Can you work these out from the model? Positions are in its coordinate system, mm. A direction names the side the tool comes from. Give positions to 0.01 mm unless a question says otherwise; leave off trailing zeros. Order: outer loops, then holes, each group sorted by start corner. A loop starts at its lowest first (then second) coordinate and runs counter-clockwise, first axis right, second up. Notation, with made-up numbers: (67.25, 33.25) - (96.25, 33.25) arc R29 ccw to (96.25, 63.25) - close; hole circle Ø8 at (61, 14.25). An arc over 180 degrees is marked (long way). Answer as a JSON object with one key per item and string values.
```python
from build123d import *

# Parameters (mm, degrees)
F0_R     = 32.6
F0_R_2   = 4.75
F1_DEPTH = 29.6
F2_R     = 2.45
F3_DEPTH = 25


with BuildPart() as f1:
    # F0 (on Front) → F1 (new body)
    with BuildSketch(Plane.XZ):
        Circle(F0_R)
        with BuildLine():
            ThreePointArc((13.747567, 17.874756), (15.860659, 16.029411), (17.728264, 13.935967))
            ThreePointArc((17.728264, 13.935967), (21.3105, 7.373268), (22.55, 0))
            ThreePointArc((22.55, 0), (22.22215, -3.831257), (21.248135, -7.55111))
            ThreePointArc((21.248135, -7.55111), (20.146089, -10.131023), (18.732227, -12.55413))
            ThreePointArc((18.732227, -12.55413), (10.343662, -20.037743), (-0.615498, -22.541598))
            ThreePointArc((-0.615498, -22.541598), (-3.409691, -22.290727), (-6.151111, -21.694846))
            ThreePointArc((-6.151111, -21.694846), (-15.860659, -16.029411), (-21.628533, -6.380364))
            ThreePointArc((-21.628533, -6.380364), (-22.253394, -3.645404), (-22.533822, -0.854022))
            ThreePointArc((-22.533822, -0.854022), (-20.146089, 10.131023), (-12.751671, 18.598317))
            ThreePointArc((-12.751671, 18.598317), (-10.343662, 20.037743), (-7.775557, 21.167031))
            ThreePointArc((-7.775557, 21.167031), (3.409691, 22.290727), (13.747567, 17.874756))
        make_face(mode=Mode.SUBTRACT)
        with BuildLine():
            ThreePointArc((-5.174181, 7.546545), (-4.197096, 8.130614), (-3.155049, 8.58884))
            Line((-3.155049, 8.58884), (-7.775557, 21.167031))
            ThreePointArc((-7.775557, 21.167031), (-10.343662, 20.037743), (-12.751671, 18.598317))
            Line((-12.751671, 18.598317), (-5.174181, 7.546545))
        make_face()
        with BuildLine():
            ThreePointArc((5.578281, 7.25295), (6.4357, 6.504173), (7.193508, 5.654727))
            Line((7.193508, 5.654727), (17.728264, 13.935967))
            ThreePointArc((17.728264, 13.935967), (15.860659, 16.029411), (13.747567, 17.874756))
            Line((13.747567, 17.874756), (5.578281, 7.25295))
        make_face()
        with BuildLine():
            Line((21.248135, -7.55111), (8.621749, -3.063976))
            ThreePointArc((8.621749, -3.063976), (8.174577, -4.110814), (7.600881, -5.094026))
            Line((7.600881, -5.094026), (18.732227, -12.55413))
            ThreePointArc((18.732227, -12.55413), (20.146089, -10.131023), (21.248135, -7.55111))
        make_face()
        with BuildLine():
            Line((-0.615498, -22.541598), (-0.249747, -9.146591))
            ThreePointArc((-0.249747, -9.146591), (-1.383533, -9.044796), (-2.495905, -8.803008))
            Line((-2.495905, -8.803008), (-6.151111, -21.694846))
            ThreePointArc((-6.151111, -21.694846), (-3.409691, -22.290727), (-0.615498, -22.541598))
        make_face()
        with BuildLine():
            ThreePointArc((-8.776101, -2.588928), (-9.029648, -1.479177), (-9.143436, -0.346532))
            Line((-9.143436, -0.346532), (-22.533822, -0.854022))
            ThreePointArc((-22.533822, -0.854022), (-22.253394, -3.645404), (-21.628533, -6.380364))
            Line((-21.628533, -6.380364), (-8.776101, -2.588928))
        make_face()
        with BuildLine():
            ThreePointArc((8.621749, -3.063976), (9.01697, -1.55459), (9.15, 0))
            ThreePointArc((9.15, 0), (8.647054, 2.991814), (7.193508, 5.654727))
            ThreePointArc((7.193508, 5.654727), (6.4357, 6.504173), (5.578281, 7.25295))
            ThreePointArc((5.578281, 7.25295), (1.383533, 9.044796), (-3.155049, 8.58884))
            ThreePointArc((-3.155049, 8.58884), (-4.197096, 8.130614), (-5.174181, 7.546545))
            ThreePointArc((-5.174181, 7.546545), (-8.174577, 4.110814), (-9.143436, -0.346532))
            ThreePointArc((-9.143436, -0.346532), (-9.029648, -1.479177), (-8.776101, -2.588928))
            ThreePointArc((-8.776101, -2.588928), (-6.4357, -6.504173), (-2.495905, -8.803008))
            ThreePointArc((-2.495905, -8.803008), (-1.383533, -9.044796), (-0.249747, -9.146591))
            ThreePointArc((-0.249747, -9.146591), (4.197096, -8.130614), (7.600881, -5.094026))
            ThreePointArc((7.600881, -5.094026), (8.174577, -4.110814), (8.621749, -3.063976))
        make_face()
        Circle(F0_R_2, mode=Mode.SUBTRACT)
        Circle(F0_R_2)
    extrude(amount=F1_DEPTH)

    # F2 (on Front) → F3 (cut, symmetric)
    with BuildSketch(Plane.XZ):
        Circle(F2_R)
    extrude(amount=F3_DEPTH, both=True, mode=Mode.SUBTRACT)


solid = f1.part
```
Q1. Which directions (+Z, -Z, +X, -X, +Y, -Y) give clear straight access to the entire face, cutting with the end or side of a thin tool? Please do faces 3 (the face through (0, -25, 0)), 4 (the face through (21.276, -14.593, 7.473)).
Recorded:
{"face 3": "+Y", "face 4": "+Y, -Y"}
Q2. If we section it at C-C, the plane z = -20: Please give me the cut outline in (x, y), then the cut area to 3 significant figures.
Recorded:
{"outline": "(-25.74, -29.6) - (-10.42, -29.6) - (-10.42, 0) - (-25.74, 0) - close; (-5.67, -29.6) - (-0.55, -29.6) - (-0.55, 0) - (-5.67, 0) - close; (10.42, -29.6) - (25.74, -29.6) - (25.74, 0) - (10.42, 0) - close", "area": "1,060 mm^2"}
Q3. If we section it at D-D, the plane y = -22.5: Please give me the cut outline in (x, z).
Recorded:
{"outline": "circle Ø65.2 at (0, 0); hole (-22.53, -0.85) - (-9.14, -0.35) arc R9.15 cw to (-5.17, 7.55) - (-12.75, 18.6) arc R22.55 ccw to start; hole (-21.63, -6.38) arc R22.55 ccw to (-6.15, -21.69) - (-2.5, -8.8) arc R9.15 cw to (-8.78, -2.59) - close; hole (-7.78, 21.17) - (-3.16, 8.59) arc R9.15 cw to (5.58, 7.25) - (13.75, 17.87) arc R22.55 ccw to start; hole circle Ø4.9 at (0, 0); hole (-0.62, -22.54) arc R22.55 ccw to (18.73, -12.55) - (7.6, -5.09) arc R9.15 cw to (-0.25, -9.15) - close; hole (7.19, 5.65) arc R9.15 cw to (9.15, 0) arc R9.15 cw to (8.62, -3.06) - (21.25, -7.55) arc R22.55 ccw to (22.55, 0) arc R22.55 ccw to (17.73, 13.94) - close"}
Q4. If we section it at B-B, the plane y = -28: Please give me the cut outline in (x, z).
Recorded:
{"outline": "circle Ø65.2 at (0, 0); hole (-22.53, -0.85) - (-9.14, -0.35) arc R9.15 cw to (-5.17, 7.55) - (-12.75, 18.6) arc R22.55 ccw to start; hole (-21.63, -6.38) arc R22.55 ccw to (-6.15, -21.69) - (-2.5, -8.8) arc R9.15 cw to (-8.78, -2.59) - close; hole (-7.78, 21.17) - (-3.16, 8.59) arc R9.15 cw to (5.58, 7.25) - (13.75, 17.87) arc R22.55 ccw to start; hole (-0.62, -22.54) arc R22.55 ccw to (18.73, -12.55) - (7.6, -5.09) arc R9.15 cw to (-0.25, -9.15) - close; hole (7.19, 5.65) arc R9.15 cw to (9.15, 0) arc R9.15 cw to (8.62, -3.06) - (21.25, -7.55) arc R22.55 ccw to (22.55, 0) arc R22.55 ccw to (17.73, 13.94) - close"}
Q5. If we section it at A-A, the plane x = 12.5: Please give me the cut outline in (y, z).
Recorded:
{"outline": "(-29.6, -30.11) - (0, -30.11) - (0, -18.77) - (-29.6, -18.77) - close; (-29.6, -8.38) - (0, -8.38) - (0, -4.44) - (-29.6, -4.44) - close; (-29.6, 9.83) - (0, 9.83) - (0, 16.25) - (-29.6, 16.25) - close; (-29.6, 18.77) - (0, 18.77) - (0, 30.11) - (-29.6, 30.11) - close"}
Q6. We'd pull the mould along X, two halves only. Please class faces 1 (the face through (0, -29.6, 0)), 2 (the face through (-8.145, -14.593, 4.168)): released by +X, released by -X, zero draft, split by the parting line, or undercut.
Recorded:
{"face 1": "zero draft", "face 2": "undercut"}
Q7. I need wall thicknesses on L1, parallel to Z at x = 0, y = -7.25; L2, parallel to X at y = -3.5, z = 6; L3, parallel to Z at x = 13.5, y = -7.25. Which ranges of each line are inside material? Lowest first, please.
Recorded:
{"L1": "z = -32.6 to -22.55, -9.15 to -2.45, 2.45 to 9.15, 22.55 to 32.6", "L2": "x = -32.04 to -21.74, -6.91 to 7.63, 21.74 to 32.04", "L3": "z = -29.67 to -18.06, -9.05 to -4.8, 10.61 to 17.55, 18.06 to 29.67"}
Q8. I'm going to push flat-ended pins straight in: pin 1 Ø5 at (x, y) = (16.5, -15.5) entering from +Z; pin 2 Ø10 at (x, y) = (-3, -7.5) entering from +Z; pin 3 Ø8 at (x, y) = (25.5, -12.5) entering from -Z. Where does each tip first touch, or does it pass through?
Recorded:
{"pin 1": "stops at z = 29.44", "pin 2": "stops at z = 32.6", "pin 3": "stops at z = -24.51"}
